Check sheet for the modelled part. Datum: model origin and axes. Units: mm. A direction names the side the tool comes from. Round coordinates to 2 decimals unless told otherwise and drop trailing zeros. Write each loop counter-clockwise with the first axis right and the second up, starting at its lowest first coordinate (ties: lowest second). Pieces come first, ordered by that corner, then holes.
from build123d import *

# Parameters (mm, degrees)
SKETCH1_R           = 1.25
BOSS_EXTRUDE1_DEPTH = 5
SKETCH2_W           = 1.75
SKETCH2_H           = 1.75
BOSS_EXTRUDE2_DEPTH = 6
BOSS_EXTRUDE3_START = -15
SKETCH3_R           = 1.25
BOSS_EXTRUDE3_DEPTH = 15


with BuildPart() as part:
    # Sketch1 → Boss-Extrude1 (new body)
    with BuildSketch(Plane.XY):
        Circle(SKETCH1_R)
    extrude(amount=BOSS_EXTRUDE1_DEPTH)

    # Sketch2 → Boss-Extrude2 (add)
    with BuildSketch(Plane.XY.offset(5)):
        Rectangle(SKETCH2_W, SKETCH2_H)
    extrude(amount=BOSS_EXTRUDE2_DEPTH)

    # Sketch3 → Boss-Extrude3 (add)
    with BuildSketch(Plane.XY.offset(BOSS_EXTRUDE3_START)):
        Circle(SKETCH3_R)
    extrude(amount=BOSS_EXTRUDE3_DEPTH)


solid = part.part
1. Sectioned sample at C-C, the plane z = -4.25. Enter the section's corners in (x, y), plus the area to 3 significant figures.
2. Sectioned sample at A-A, the plane y = 0. Enter the section's corners in (x, z) (3 decimals).
3. Go/stop test with flat-tipped pins: pin 1 (1.4 mm diameter, centred on x = 0, z = 7.5, fed in from -Y) (3 decimals); pin 2 (0.9 mm diameter, centred on y = 0, z = 8, fed in from +X) (3 decimals). Record where each tip stops, or that it passes through.
4. Sectioned sample at D-D, the plane z = 6. Enter the section's corners in (x, y) (3 decimals).
5. Set-up check for faces 1 (the flat face through (0, -0.875, 8)), 2 (the flat face through (0.875, 0, 8)), 3 (the flat face through (0, 0.875, 8)): record each of +Z, -Z, +X, -X, +Y, -Y from which the full face is reachable in a straight line by a thin tool's end or side.
6. Scan lines: line 1 along X through (y, z) = (0.05, -0.5); line 2 along Z through (x, y) = (0.95, -0.6); line 3 along Y through (x, z) = (-0.1, 5.25) (3 decimals). Record each from-to range of solid material in increasing order.
Computed values:
1. outline: circle Ø2.5 at (0, 0)
1. area: 4.91 mm2
2. outline: (-1.25, -15) - (1.25, -15) - (1.25, 5) - (0.875, 5) - (0.875, 11) - (-0.875, 11) - (-0.875, 5) - (-1.25, 5) - close
3. pin 1: stops at y = -0.875
3. pin 2: stops at x = 0.875
4. outline: (-0.875, -0.875) - (0.875, -0.875) - (0.875, 0.875) - (-0.875, 0.875) - close
5. face 1: +Z, +X, -X, -Y
5. face 2: +Z, +X, +Y, -Y
5. face 3: +Z, +X, -X, +Y
6. line 1: x = -1.25 to 1.25
6. line 2: z = -15 to 5
6. line 3: y = -0.875 to 0.875
